Read the model definition and answer for the solid it produces. Units are mm, in the model's axes. A direction names the side the tool comes from. Coordinates: 2 decimals unless noted, no trailing zeros. Loops run counter-clockwise (first coordinate to the right, second up) from the corner with the lowest first, then second, coordinate; pieces in that order, holes last. Notation, with made-up numbers: (-20.5, 43.25) -> (-8.5, 43.25) arc R25 ccw to (-8.5, 70.25) -> close; hole circle Ø10 at (-25.5, 13.5). An arc over 180 degrees is marked (long way). Answer as CSV lines item,"result".
```python
from build123d import *

# Parameters (mm, degrees)
SKETCH_2_W                    = 62
SKETCH_2_H                    = 62
SKETCH_2_R                    = 21
EXTRUDE_2_DEPTH               = 220
SKETCH_4_R                    = 21
SKETCH_4_R_2                  = 3.5
EXTRUDE_3_DEPTH               = 5
CUT_EXTRUDE_1_DEPTH           = 40
HOLE_WIZARD_M10_1_D           = 8.5
HOLE_WIZARD_M10_1_CSINK_D     = 10.05
HOLE_WIZARD_M10_1_CSINK_ANGLE = 90
SKETCH_7_W                    = 10
SKETCH_7_H                    = 80
CUT_EXTRUDE_2_DEPTH           = 5
SKETCH_10_W                   = 10
SKETCH_10_H                   = 80
CUT_EXTRUDE_3_DEPTH           = 5


with BuildPart() as part:
    # 草图2 → 凸台-拉伸2 (new body)
    with BuildSketch(Plane(origin=(0, 0, 0), x_dir=(1, 0, 0), z_dir=(0, 1, 0))):
        Rectangle(SKETCH_2_W, SKETCH_2_H)
        with Locations(Location((0, 0, 0), (0, 0, 270))):
            Circle(SKETCH_2_R, mode=Mode.SUBTRACT)
    extrude(amount=EXTRUDE_2_DEPTH)

    # 草图4 → 凸台-拉伸3 (add)
    with BuildSketch(Plane.XZ):
        with Locations(Location((0, 0, 0), (0, 0, 270))):
            Circle(SKETCH_4_R)
        with Locations(Location((0, 0, 0), (0, 0, 270))):
            Circle(SKETCH_4_R_2, mode=Mode.SUBTRACT)
    extrude(amount=-EXTRUDE_3_DEPTH)

    # 草图3 → 切除-拉伸1 (cut, symmetric)
    with BuildSketch(Plane(origin=(0, 110, 0), x_dir=(1, 0, 0), z_dir=(0, 1, 0))):
        Polygon((-21, 0), (-21, 36.73556218), (47.200279586, 36.73556218), (47.200279586, -37.147800903), (-21, -37.147800903), align=None)
    extrude(amount=CUT_EXTRUDE_1_DEPTH, both=True, mode=Mode.SUBTRACT)

    # M10 螺纹孔1 (through all)
    with Locations(Plane(origin=(-21, 110, 0), x_dir=(0, 0, 1), z_dir=(1, 0, 0))):
        with Locations((0, 0)):
            CounterSinkHole(HOLE_WIZARD_M10_1_D / 2, HOLE_WIZARD_M10_1_CSINK_D / 2, counter_sink_angle=HOLE_WIZARD_M10_1_CSINK_ANGLE)

    # 草图7 → 切除-拉伸2 (cut)
    with BuildSketch(Plane(origin=(-21, 0, 0), x_dir=(0, 0, -1), z_dir=(1, 0, 0))):
        with Locations((21, 110)):
            Rectangle(SKETCH_7_W, SKETCH_7_H)
    extrude(amount=-CUT_EXTRUDE_2_DEPTH, mode=Mode.SUBTRACT)

    # 草图10 → 切除-拉伸3 (cut)
    with BuildSketch(Plane(origin=(-21, 0, 0), x_dir=(0, 0, -1), z_dir=(1, 0, 0))):
        with Locations((-21, 110)):
            Rectangle(SKETCH_10_W, SKETCH_10_H)
    extrude(amount=-CUT_EXTRUDE_3_DEPTH, mode=Mode.SUBTRACT)


solid = part.part
```
Q1. Find the intervals of material crossed by probe 1 along Y at (x, z) = (-21, -21); probe 2 along Z at (x, y) = (-27.25, 110); probe 3 along X at (y, z) = (40, 0), in increasing order. Write a range as [from, to].
Results:
probe 1,"y = [0, 70], [150, 220]"
probe 2,"z = [-31, -4.25], [4.25, 31]"
probe 3,"x = [-31, -21], [21, 31]"
Q2. Given pin 1 Ø3 at (y, z) = (106, -21) entering from +X; pin 2 Ø17 at (x, z) = (-1.5, 6.5) entering from +Y; pin 3 Ø4 at (y, z) = (106, -28.5) entering from +X, each flat-ended and moving along its own axis, determine where each tip first touches the part or whether it passes through.
Results:
pin 1,"stops at x = -26"
pin 2,"stops at y = 5"
pin 3,"stops at x = -21"
Q3. A cutting plane is placed at C-C, the plane z = -8.5. Write down the section's boundary in (x, y), and give its area (3 significant figures).
Results:
outline,"(-31, 0) -> (31, 0) -> (31, 70) -> (19.2, 70) -> (19.2, 5) -> (-19.2, 5) -> (-19.2, 70) -> (-21, 70) -> (-21, 150) -> (-19.2, 150) -> (-19.2, 220) -> (-31, 220) -> close; (19.2, 150) -> (31, 150) -> (31, 220) -> (19.2, 220) -> close"
area,"4,300 mm²"
Q4. For faces 4 (the face through (6.31, 184.51, 20.03)), 5 (the face through (-23, 109, -16)), 6 (the face through (-21, 111, -29)), determine the directions among +Z, -Z, +X, -X, +Y, -Y from which every point of the face is accessible in a straight line to the end or side of a thin tool.
Results:
face 4,"+Y"
face 5,"+X"
face 6,"+Z, -Z, +X"
Q5. A cutting plane is placed at B-B, the plane y = 110. Write down the section's boundary in (x, z) (3 decimals), and give its area (3 significant figures).
Results:
outline,"(-31, -31) -> (-21, -31) -> (-21, -26) -> (-26, -26) -> (-26, -16) -> (-21, -16) -> (-21, -5.025) -> (-21.775, -4.25) -> (-31, -4.25) -> close; (-31, 4.25) -> (-21.775, 4.25) -> (-21, 5.025) -> (-21, 16) -> (-26, 16) -> (-26, 26) -> (-21, 26) -> (-21, 31) -> (-31, 31) -> close"
area,"434 mm²"
Q6. A cutting plane is placed at A-A, the plane x = 0. Write down the section's boundary in (y, z), and give its area (4 significant figures).
Results:
outline,"(0, -31) -> (70, -31) -> (70, -21) -> (5, -21) -> (5, -3.5) -> (0, -3.5) -> close; (0, 3.5) -> (5, 3.5) -> (5, 21) -> (70, 21) -> (70, 31) -> (0, 31) -> close; (150, -31) -> (220, -31) -> (220, -21) -> (150, -21) -> close; (150, 21) -> (220, 21) -> (220, 31) -> (150, 31) -> close"
area,"2,975 mm²"
Q7. A cutting plane is placed at D-D, the plane y = 58.5. Write down the section's boundary in (x, z).
Results:
outline,"(-31, -31) -> (31, -31) -> (31, 31) -> (-31, 31) -> close; hole circle Ø42 at (0, 0)"
Q8. For a pull along Z with two mould halves and no side action, classify faces 1 (the face through (6.31, 37.04, 20.03)), 2 (the face through (-28, 108, -31)), 3 (the face through (-21, 111, 28)) as pulls with the +Z half, pulls with the -Z half, needs draft (parallel to the pull), parting line crosses it, or undercut.
Results:
face 1,"undercut"
face 2,"pulls with the -Z half"
face 3,"needs draft"
